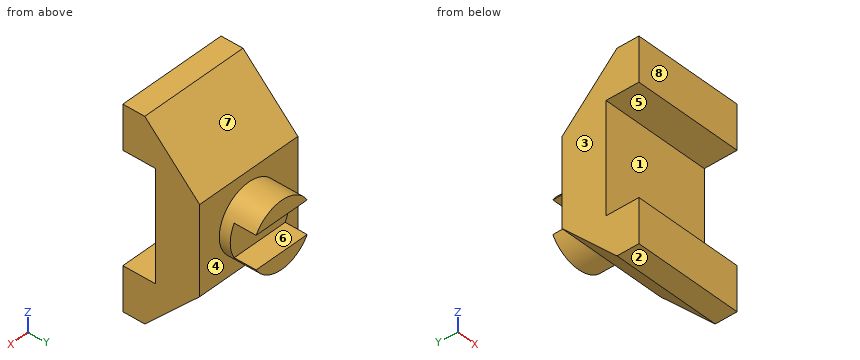
```python
from build123d import *

# Parameters (mm, degrees)
SALIENTE_EXTRUIR1_DEPTH                = 25
CORTAR_EXTRUIR1_REACH                  = 73.764
CORTAR_EXTRUIR1_END_RADIUS             = 15
CROQUIS5_W                             = 15
CROQUIS5_H                             = 10
CORTAR_EXTRUIR1_DIRECTION_2_REACH      = 73.764
CORTAR_EXTRUIR1_DIRECTION_2_END_RADIUS = 15


with BuildPart() as part:
    # Croquis2 → Saliente-Extruir1 (new, symmetric)
    with BuildSketch(Plane(origin=(0, 0, 0), x_dir=(0, 0, -1), z_dir=(1, 0, 0))):
        Polygon((-45, 0), (-25, 0), (-25, 15), (25, 15), (25, 0), (45, 0), (45, 10), (20, 35), (-20, 35), (-45, 10), align=None)
    extrude(amount=SALIENTE_EXTRUIR1_DEPTH, both=True)

    # Croquis3 → Revolución2 (revolve)
    with BuildSketch(Plane(origin=(0, 0, 0), x_dir=(0, 0, -1), z_dir=(1, 0, 0))):
        Polygon((0, 35), (15, 35), (15, 50), (7.5, 50), (7.5, 40), (0, 40), align=None)
    revolve(axis=Axis((0, -6.406995379, 0), (0, 1, 0)))

    # Cortar-Extruir1: up to this cylinder (the profile starts inside it)
    cortar_extruir1_end = Plane(origin=(0, 45, 0), z_dir=(0, -1, 0)) * Cylinder(CORTAR_EXTRUIR1_END_RADIUS, 178.528, mode=Mode.PRIVATE)
    # Croquis5 → Cortar-Extruir1 (cut, up to the surface)
    with BuildSketch(Plane(origin=(0, 0, 0), x_dir=(0, 0, -1), z_dir=(1, 0, 0)), mode=Mode.PRIVATE) as cortar_extruir1_sk1:
        with Locations((0, 45)):
            Rectangle(CROQUIS5_W, CROQUIS5_H)
    cortar_extruir1_tool1 = extrude(cortar_extruir1_sk1.sketch, amount=-CORTAR_EXTRUIR1_REACH, mode=Mode.PRIVATE) & cortar_extruir1_end
    add(cortar_extruir1_tool1.solids().sort_by_distance((0, 45, 0))[0], mode=Mode.SUBTRACT)

    # Cortar-Extruir1 direction 2: up to this cylinder (the profile starts inside it)
    cortar_extruir1_direction_2_end = Plane(origin=(0, 45, 0), z_dir=(0, -1, 0)) * Cylinder(CORTAR_EXTRUIR1_DIRECTION_2_END_RADIUS, 178.528, mode=Mode.PRIVATE)
    # Croquis5 → Cortar-Extruir1 direction 2 (cut, up to the surface)
    with BuildSketch(Plane(origin=(0, 0, 0), x_dir=(0, 0, -1), z_dir=(1, 0, 0)), mode=Mode.PRIVATE) as cortar_extruir1_direction_2_sk1:
        with Locations((0, 45)):
            Rectangle(CROQUIS5_W, CROQUIS5_H)
    cortar_extruir1_direction_2_tool1 = extrude(cortar_extruir1_direction_2_sk1.sketch, amount=CORTAR_EXTRUIR1_DIRECTION_2_REACH, mode=Mode.PRIVATE) & cortar_extruir1_direction_2_end
    add(cortar_extruir1_direction_2_tool1.solids().sort_by_distance((0, 45, 0))[0], mode=Mode.SUBTRACT)


solid = part.part
```
The listing builds one solid part. Answer for the finished solid, in the listing's coordinates (mm). Face numbers are marked on the shaded views. A direction names the side the tool comes from. Coordinates: 2 decimals unless noted, no trailing zeros. Loops run counter-clockwise (first coordinate to the right, second up) from the corner with the lowest first, then second, coordinate; pieces in that order, holes last. Notation, with made-up numbers: (49, 66.25) -> (69, 66.25) arc R20 cw to (69, 98.25) -> close; hole circle Ø7 at (-15, 4). An arc over 180 degrees is marked (long way). Return JSON: item names as keys, results as strings. Group by question number.
(1) A cutting plane is placed at C-C on z = 0. Write down the section's boundary in (x, y).
(2) A cutting plane is placed at A-A on y = 9. Write down the section's boundary in (x, z), and give its area (3 significant figures).
(3) Determine the mould class of the marked faces 1, 2 and 3 for opening direction Z: released by +Z, released by -Z, zero draft, split by the parting line, or undercut.
(4) Given pin 1 Ø6 at (x, y) = (-18, 30.5) entering from +Z; pin 2 Ø15 at (x, z) = (-8.5, 2) entering from -Y; pin 3 Ø7.5 at (x, z) = (-4.5, 3) entering from +Y, each flat-ended and moving along its own axis, determine where each tip first touches the part or whether it passes through.
(5) A cutting plane is placed at D-D on y = 14. Write down the section's boundary in (x, z), and give its area (3 significant figures).
(6) A cutting plane is placed at B-B on x = -19.5. Write down the section's boundary in (y, z).
(7) Find the intervals of material crossed by probe 1 along Z at (x, y) = (-13, 9); probe 2 along Y at (x, z) = (21, 0); probe 3 along Y at (x, z) = (-3, 3.5), in increasing order. Write a range as from..to.
(8) Which of the six approach directions +Z, -Z, +X, -X, +Y, -Y give full straight-line access (tool end or side, diameter ignored) to the marked faces 4, 5, 6, 7 and 8?
The answers:
{
 "1": {"outline": "(-25, 15) -> (25, 15) -> (25, 35) -> (15, 35) -> (15, 40) -> (-15, 40) -> (-15, 35) -> (-25, 35) -> close"},
 "2": {"outline": "(-25, -45) -> (25, -45) -> (25, -25) -> (-25, -25) -> close; (-25, 25) -> (25, 25) -> (25, 45) -> (-25, 45) -> close", "area": "2,000 mm^2"},
 "3": {"face 1": "undercut", "face 2": "released by -Z", "face 3": "zero draft"},
 "4": {"pin 1": "stops at z = 27.5", "pin 2": "stops at y = 15", "pin 3": "stops at y = 40"},
 "5": {"outline": "(-25, -41) -> (25, -41) -> (25, -25) -> (-25, -25) -> close; (-25, 25) -> (25, 25) -> (25, 41) -> (-25, 41) -> close", "area": "1,600 mm^2"},
 "6": {"outline": "(0, -45) -> (10, -45) -> (35, -20) -> (35, 20) -> (10, 45) -> (0, 45) -> (0, 25) -> (15, 25) -> (15, -25) -> (0, -25) -> close"},
 "7": {"probe 1": "z = -45..-25, 25..45", "probe 2": "y = 15..35", "probe 3": "y = 15..40"},
 "8": {"face 4": "+Y", "face 5": "+X, -X, -Y", "face 6": "+X, -X, +Y", "face 7": "+Z, +X, -X, +Y", "face 8": "+Z, -Z, +X, -X, -Y"}
}
